Verification items for the finished model (mm, model axes). A direction names the side the tool comes from. Round coordinates to 2 decimals unless told otherwise and drop trailing zeros. Order: outer loops, then holes, each group sorted by start corner. A loop starts at its lowest first (then second) coordinate and runs counter-clockwise, first axis right, second up. Notation, with made-up numbers: (47.25, 25) -> (69.25, 25) arc R33 ccw to (69.25, 57) -> close; hole circle Ø5 at (88, 38). An arc over 180 degrees is marked (long way). Return JSON: item names as keys, results as strings. Group by question number.
1) Draft check along X on faces 6 (the cylindrical face through (-18.14, 1.52, -6.6)), 7 (the flat face through (0, 10, 0)), 8 (the flat face through (1, 18, 0)). Enter one of: pulls with the +X half, pulls with the -X half, needs draft (parallel to the pull), parting line crosses it, or undercut.
2) Section check C-C on y = 13. Enter the section's corners in (x, z), plus the area to 3 significant figures.
3) Section check D-D on y = 6. Enter the section's corners in (x, z).
4) Section check B-B on x = 8. Enter the section's corners in (y, z).
5) Tool access check on faces 1 (the cylindrical face through (-18.1, 1.52, 6.64)), 2 (the cylindrical face through (1.48, 17.1, -6.64)), 3 (the flat face through (8, 3, -2)), 4 (the flat face through (-3, 3, 0)), 5 (the flat face through (-9, 10, 0)). Record the directions out of +Z, -Z, +X, -X, +Y, -Y that give a thin tool (end or side, any length) a straight path to the whole face; none if there is none.
6) Scan lines: L1, parallel to X at y = 2.25, z = 0; L2, parallel to X at y = 9.5, z = -2.25; L3, parallel to Y at x = -7.9, z = 0. Record each from-to range of solid material in increasing order.
7) Section check A-A on z = 0. Enter the section's corners in (x, y).
8) Depth check by flat-ended pin: pin 1 (7.5 mm diameter, centred on y = 13.5, z = 0, fed in from -X); pin 2 (2.5 mm diameter, centred on y = 13, z = 0, fed in from -X); pin 3 (1.5 mm diameter, centred on x = -14, z = -5.5, fed in from +Y); pin 4 (2 mm diameter, centred on y = 7, z = 5.5, fed in from +X). Enter the tip coordinate at first touch or a pass-through.
```python
from build123d import *

# Parameters (mm, degrees)
CROQUIS1_W              = 38
CROQUIS1_H              = 15
SALIENTE_EXTRUIR1_DEPTH = 3
CROQUIS2_W              = 3
CROQUIS2_H              = 15
SALIENTE_EXTRUIR2_DEPTH = 15
CROQUIS3_W              = 6
CROQUIS3_H              = 15
CORTAR_EXTRUIR1_DEPTH   = 15
CORTAR_EXTRUIR2_DEPTH   = 15
CORTAR_EXTRUIR3_DEPTH   = 15
CROQUIS6_R              = 1.5
CORTAR_EXTRUIR4_DEPTH   = 15
CROQUIS7_R              = 1.5
CORTAR_EXTRUIR5_DEPTH   = 15


with BuildPart() as part:
    # Croquis1 → Saliente-Extruir1 (new body)
    with BuildSketch(Plane(origin=(0, 0, 0), x_dir=(1, 0, 0), z_dir=(0, 1, 0))):
        Rectangle(CROQUIS1_W, CROQUIS1_H)
    extrude(amount=SALIENTE_EXTRUIR1_DEPTH)

    # Croquis2 → Saliente-Extruir2 (add)
    with BuildSketch(Plane(origin=(0, 3, 0), x_dir=(1, 0, 0), z_dir=(0, 1, 0))):
        with Locations((-7.5, 0)):
            Rectangle(CROQUIS2_W, CROQUIS2_H)
        with Locations((1.5, 0)):
            Rectangle(CROQUIS2_W, CROQUIS2_H)
    extrude(amount=SALIENTE_EXTRUIR2_DEPTH)

    # Croquis3 → Cortar-Extruir1 (cut)
    with BuildSketch(Plane(origin=(0, 3, 0), x_dir=(1, 0, 0), z_dir=(0, 1, 0))):
        with Locations((16, 0)):
            Rectangle(CROQUIS3_W, CROQUIS3_H)
    extrude(amount=-CORTAR_EXTRUIR1_DEPTH, mode=Mode.SUBTRACT)

    # Croquis4 → Cortar-Extruir2 (cut)
    with BuildSketch(Plane(origin=(0, 3, 0), x_dir=(1, 0, 0), z_dir=(0, 1, 0))):
        with BuildLine():
            Line((-19, 7.5), (-19, 4.5))
            ThreePointArc((-19, 4.5), (-18.121320344, 6.621320344), (-16, 7.5))
            Line((-16, 7.5), (-19, 7.5))
        make_face()
        with BuildLine():
            ThreePointArc((-16, -7.5), (-18.121320344, -6.621320344), (-19, -4.5))
            Line((-19, -4.5), (-19, -7.5))
            Line((-19, -7.5), (-16, -7.5))
        make_face()
        with BuildLine():
            Line((13, -4.5), (13, -7.5))
            Line((13, -7.5), (10, -7.5))
            ThreePointArc((10, -7.5), (12.121320344, -6.621320344), (13, -4.5))
        make_face()
        with BuildLine():
            Line((10, 7.5), (13, 7.5))
            Line((13, 7.5), (13, 4.5))
            ThreePointArc((13, 4.5), (12.121320344, 6.621320344), (10, 7.5))
        make_face()
    extrude(amount=-CORTAR_EXTRUIR2_DEPTH, mode=Mode.SUBTRACT)

    # Croquis5 → Cortar-Extruir3 (cut)
    with BuildSketch(Plane.ZY.offset(9)):
        with BuildLine():
            Line((-4.5, 18), (-7.5, 18))
            Line((-7.5, 18), (-7.5, 15))
            ThreePointArc((-7.5, 15), (-6.621320344, 17.121320344), (-4.5, 18))
        make_face()
        with BuildLine():
            Line((4.5, 18), (7.5, 18))
            Line((7.5, 18), (7.5, 15))
            ThreePointArc((7.5, 15), (6.621320344, 17.121320344), (4.5, 18))
        make_face()
    extrude(amount=-CORTAR_EXTRUIR3_DEPTH, mode=Mode.SUBTRACT)

    # Croquis6 → Cortar-Extruir4 (cut)
    with BuildSketch(Plane.ZY.offset(9)):
        with Locations((0, 13)):
            Circle(CROQUIS6_R)
    extrude(amount=-CORTAR_EXTRUIR4_DEPTH, mode=Mode.SUBTRACT)

    # Croquis7 → Cortar-Extruir5 (cut)
    with BuildSketch(Plane(origin=(0, 3, 0), x_dir=(1, 0, 0), z_dir=(0, 1, 0))):
        with Locations(Location((-14, 0, 0), (0, 0, 270))):
            Circle(CROQUIS7_R)
        with Locations(Location((8, 0, 0), (0, 0, 270))):
            Circle(CROQUIS7_R)
    extrude(amount=-CORTAR_EXTRUIR5_DEPTH, mode=Mode.SUBTRACT)


solid = part.part
```
Check result:
{
 "1": {"face 6": "pulls with the -X half", "face 7": "undercut", "face 8": "needs draft"},
 "2": {"outline": "(-9, -7.5) -> (-6, -7.5) -> (-6, -1.5) -> (-9, -1.5) -> close; (-9, 1.5) -> (-6, 1.5) -> (-6, 7.5) -> (-9, 7.5) -> close; (0, -7.5) -> (3, -7.5) -> (3, -1.5) -> (0, -1.5) -> close; (0, 1.5) -> (3, 1.5) -> (3, 7.5) -> (0, 7.5) -> close", "area": "72.0 mm^2"},
 "3": {"outline": "(-9, -7.5) -> (-6, -7.5) -> (-6, 7.5) -> (-9, 7.5) -> close; (0, -7.5) -> (3, -7.5) -> (3, 7.5) -> (0, 7.5) -> close"},
 "4": {"outline": "(0, -7.5) -> (3, -7.5) -> (3, -1.5) -> (0, -1.5) -> close; (0, 1.5) -> (3, 1.5) -> (3, 7.5) -> (0, 7.5) -> close"},
 "5": {"face 1": "+Z, -X, +Y, -Y", "face 2": "-Z, +X, -X, +Y", "face 3": "+Z, -Z, +X, +Y", "face 4": "+Z, -Z, +Y", "face 5": "+Z, -Z, -X, +Y"},
 "6": {"L1": "-19 to -15.5, -12.5 to 6.5, 9.5 to 13", "L2": "-9 to -6, 0 to 3", "L3": "0 to 11.5, 14.5 to 18"},
 "7": {"outline": "(-19, 0) -> (-15.5, 0) -> (-15.5, 3) -> (-19, 3) -> close; (-12.5, 0) -> (6.5, 0) -> (6.5, 3) -> (3, 3) -> (3, 11.5) -> (0, 11.5) -> (0, 3) -> (-6, 3) -> (-6, 11.5) -> (-9, 11.5) -> (-9, 3) -> (-12.5, 3) -> close; (-9, 14.5) -> (-6, 14.5) -> (-6, 18) -> (-9, 18) -> close; (0, 14.5) -> (3, 14.5) -> (3, 18) -> (0, 18) -> close; (9.5, 0) -> (13, 0) -> (13, 3) -> (9.5, 3) -> close"},
 "8": {"pin 1": "x = -9", "pin 2": "through", "pin 3": "y = 3", "pin 4": "x = 3"}
}
